Here's how the part is built. I have some questions about the finished solid (model axes, mm). A direction names the side the tool comes from. Round coordinates to 2 decimals unless told otherwise and drop trailing zeros. Write each loop counter-clockwise with the first axis right and the second up, starting at its lowest first coordinate (ties: lowest second). Pieces come first, ordered by that corner, then holes. Notation, with made-up numbers: (47.25, -9.5) -> (61.25, -9.5) arc R19 ccw to (61.25, 11.5) -> close; hole circle Ø1 at (71.5, 45). An arc over 180 degrees is marked (long way). Answer as CSV lines item,"result".
from build123d import *

# Parameters (mm, degrees)
BOSS_EXTRUDE2_DEPTH = 19.6
CHAMFER1_SIZE       = 3.184213023
CHAMFER1_SIZE_2     = 9.8
CHAMFER2_SIZE       = 9.8
CHAMFER2_SIZE_2     = 0.427877241


with BuildPart() as part:
    # Sketch4 → Boss-Extrude2 (new body)
    with BuildSketch(Plane.XY):
        with BuildLine():
            Line((14.247619048, -73.430547809), (216.628571429, -34.162875184))
            ThreePointArc((216.628571429, -34.162875184), (244.8, 0), (216.628571429, 34.162875184))
            Line((216.628571429, 34.162875184), (14.247619048, 73.430547809))
            ThreePointArc((14.247619048, 73.430547809), (-74.8, 0), (14.247619048, -73.430547809))
        make_face()
        with BuildLine():
            Line((12.380952381, 63.809968016), (214.761904762, 24.542295391))
            ThreePointArc((214.761904762, 24.542295391), (235, 0), (214.761904762, -24.542295391))
            Line((214.761904762, -24.542295391), (12.380952381, -63.809968016))
            ThreePointArc((12.380952381, -63.809968016), (-65, 0), (12.380952381, 63.809968016))
        make_face(mode=Mode.SUBTRACT)
    extrude(amount=BOSS_EXTRUDE2_DEPTH)

    # Chamfer1
    # the kernel refuses this chamfer: 9.8, 3.184213023 mm, written as the material it takes off along each edge
    with BuildSketch(Plane(origin=(0, 0, 19.6), x_dir=(0.19047619047619063, -0.9816918156232525, 0), z_dir=(0.9816918156232525, 0.19047619047619063, 0))) as chamfer1_piece_1:
        Polygon((65, CHAMFER1_SIZE), (65 + CHAMFER1_SIZE_2, 0), (65, 0), align=None)
    revolve(axis=Axis((0, 0, 19.6), (0, 0, -1)), revolution_arc=201.961150855, mode=Mode.SUBTRACT)
    with BuildSketch(Plane(origin=(214.761904762, -24.542295391, 19.6), x_dir=(-0.021348671206160026, 0.1100285329369752, -0.9936991275921844), z_dir=(-0.9816918156232526, -0.1904761904761905, 0)), Plane(origin=(12.380952381, 63.809968016, 19.6), x_dir=(-0.021348671206159867, -0.1100285329369744, -0.9936991275921844), z_dir=(0.9816918156232526, -0.1904761904761905, 0))) as chamfer1_piece_2:
        Polygon((CHAMFER1_SIZE * 0.993699127618, CHAMFER1_SIZE * 0.112080523835), (-CHAMFER1_SIZE_2 * 0.112080523832, CHAMFER1_SIZE_2 * 0.993699127592), (0, 0), align=None)
    extrude(amount=206.155281281, mode=Mode.SUBTRACT)
    with BuildSketch(Plane(origin=(210, 0, 19.6), x_dir=(0.19047619047619035, 0.9816918156232525, 0), z_dir=(-0.9816918156232525, 0.19047619047619035, 0))) as chamfer1_piece_3:
        Polygon((25, CHAMFER1_SIZE), (25 + CHAMFER1_SIZE_2, 0), (25, 0), align=None)
    revolve(axis=Axis((210, 0, 19.6), (0, 0, -1)), revolution_arc=158.038849145, mode=Mode.SUBTRACT)

    # Chamfer2
    # the kernel refuses this chamfer: 9.8, 0.427877241 mm, written as the material it takes off along each edge
    with BuildSketch(Plane(origin=(0, 0, 0), x_dir=(0.19047619047619063, -0.9816918156232525, 0), z_dir=(0.9816918156232525, 0.19047619047619063, 0))) as chamfer2_piece_1:
        Polygon((65 + CHAMFER2_SIZE, 0), (65, -CHAMFER2_SIZE_2 * 0.999999998839), (65, 0), align=None)
    revolve(axis=Axis((0, 0, 0), (0, 0, -1)), revolution_arc=201.961150855, mode=Mode.SUBTRACT)
    with BuildSketch(Plane(origin=(214.761904762, -24.542295391, 0), x_dir=(0.1904759224026141, -0.9816904340036641, -0.0016777278000430975), z_dir=(-0.9816918156232526, -0.1904761904761905, 0)), Plane(origin=(12.380952381, 63.809968016, 0), x_dir=(0.19047592240261413, 0.9816904340036641, -0.0016777278000430988), z_dir=(0.9816918156232526, -0.1904761904761905, 0))) as chamfer2_piece_2:
        Polygon((CHAMFER2_SIZE * 0.999998592614, CHAMFER2_SIZE * 0.00167772780004), (-CHAMFER2_SIZE_2 * 0.0016777277981, CHAMFER2_SIZE_2 * 0.999998591453), (0, 0), align=None)
    extrude(amount=206.155281281, mode=Mode.SUBTRACT)
    with BuildSketch(Plane(origin=(210, 0, 0), x_dir=(0.19047619047619035, 0.9816918156232525, 0), z_dir=(-0.9816918156232525, 0.19047619047619035, 0))) as chamfer2_piece_3:
        Polygon((25 + CHAMFER2_SIZE, 0), (25, -CHAMFER2_SIZE_2 * 0.999999998839), (25, 0), align=None)
    revolve(axis=Axis((210, 0, 0), (0, 0, -1)), revolution_arc=158.038849145, mode=Mode.SUBTRACT)


solid = part.part
Item 1: For faces 1 (the flat face through (115, -43.9, 8.3)), 2 (the conical face through (235.608, 0.495, 16.615)), 3 (the conical face through (-65.456, -1.615, 0.407)), 4 (the flat face through (116.855, 53.522, 9.663)), which set-ups out of +Z, -Z, +X, -X, +Y, -Y let a thin tool reach every point of the face, with its end or its side?
Results found:
face 1,"+Z, -Z"
face 2,"+Z"
face 3,"-Z"
face 4,"+Z, -Z, +X, +Y"
Item 2: I need wall thicknesses on L1, parallel to X at y = 0, z = 12; L2, parallel to Y at x = 0, z = 5; L3, parallel to X at y = -22.5, z = 11.5. Which ranges of each line are inside material? Lowest first, please.
Results found:
L1,"x = -74.8 to -65, 235 to 244.8"
L2,"y = -74.8 to -65, 65 to 74.8"
L3,"x = -71.34 to -60.98, 220.9 to 236.55"
Item 3: If we mould it in two halves opening along Y, with no side actions, what happens to faces 5 (the flat face through (112.15, 44.45, 8.31)), 6 (the flat face through (114.02, -54.07, 9.66)), 7 (the cylindrical face through (-74.777, 1.845, 9.663))? For each: pulls with the +Y half, pulls with the -Y half, needs draft (parallel to the pull), parting line crosses it, or undercut.
Results found:
face 5,"undercut"
face 6,"pulls with the -Y half"
face 7,"parting line crosses it"
Item 4: Will these pins go through, and if not, where does the flat tip stop? pin 1 (3 mm diameter, centred on x = 204.5, z = 14, fed in from -Y); pin 2 (4 mm diameter, centred on y = 11.5, z = 12, fed in from -X); pin 3 (1 mm diameter, centred on y = 15, z = 16.5, fed in from +X).
Results found:
pin 1,"stops at y = -36.81"
pin 2,"stops at x = -74.19"
pin 3,"stops at x = 241.64"
Item 5: Suppose I cut it at C-C, the plane x = 0. List the corners of the cut face in (y, z) for me.
Results found:
outline,"(-74.8, 0) -> (-65, 0.43) -> (-65, 16.42) -> (-74.8, 19.6) -> close; (65, 0.43) -> (74.8, 0) -> (74.8, 19.6) -> (65, 16.42) -> close"
Item 6: Suppose I cut it at B-B, the plane z = 6.25. List the corners of the cut face in (x, y) for me.
Results found:
outline,"(14.25, -73.43) -> (216.63, -34.16) arc R34.8 ccw to (216.63, 34.16) -> (14.25, 73.43) arc R74.8 ccw (long way) to start; hole (12.38, -63.81) -> (214.76, -24.54) arc R25 ccw to (214.76, 24.54) -> (12.38, 63.81) arc R65 ccw (long way) to start"
Item 7: Suppose I cut it at A-A, the plane y = 0. List the corners of the cut face in (x, z) for me, then the cut area to 3 significant figures.
Results found:
outline,"(-74.8, 0) -> (-65, 0.43) -> (-65, 16.42) -> (-74.8, 19.6) -> close; (235, 0.43) -> (244.8, 0) -> (244.8, 19.6) -> (235, 16.42) -> close"
area,"349 mm²"
